from build123d import *

# Parameters (mm, degrees)
SKETCH1_R           = 1.5
SKETCH1_R_2         = 1
SKETCH1_R_3         = 0.5
BOSS_EXTRUDE1_DEPTH = 1.6
BOSS_EXTRUDE2_START = 1.6
SKETCH2_W           = 8
SKETCH2_H           = 8
BOSS_EXTRUDE2_DEPTH = 4.4
SKETCH3_W           = 10
SKETCH3_H           = 2.75
BOSS_EXTRUDE3_DEPTH = 3
SKETCH4_W           = 6.75
SKETCH4_H           = 6.75
SKETCH4_W_2         = 3
SKETCH4_H_2         = 3
SKETCH4_H_3         = 4
SKETCH4_W_3         = 1.5
BOSS_EXTRUDE4_DEPTH = 1.5


with BuildPart() as part:
    # Sketch1 → Boss-Extrude1 (new body)
    with BuildSketch(Plane(origin=(0, 0, 0), x_dir=(1, 0, 0), z_dir=(0, 1, 0))):
        with BuildLine():
            Line((-10, 28), (-10, 27))
            ThreePointArc((-10, 27), (-10.585786438, 25.585786438), (-12, 25))
            Line((-12, 25), (-15, 25))
            ThreePointArc((-15, 25), (-22.071067812, 22.071067812), (-25, 15))
            Line((-25, 15), (-25, -15))
            ThreePointArc((-25, -15), (-22.071067812, -22.071067812), (-15, -25))
            Line((-15, -25), (15, -25))
            ThreePointArc((15, -25), (22.071067812, -22.071067812), (25, -15))
            Line((25, -15), (25, 15))
            ThreePointArc((25, 15), (22.071067812, 22.071067812), (15, 25))
            Line((15, 25), (12, 25))
            ThreePointArc((12, 25), (10.585786438, 25.585786438), (10, 27))
            Line((10, 27), (10, 28))
            ThreePointArc((10, 28), (9.414213562, 29.414213562), (8, 30))
            Line((8, 30), (6, 30))
            Line((6, 30), (6, 27))
            ThreePointArc((6, 27), (4, 25), (2, 27))
            Line((2, 27), (2, 30))
            Line((2, 30), (-2, 30))
            Line((-2, 30), (-2, 27))
            ThreePointArc((-2, 27), (-4, 25), (-6, 27))
            Line((-6, 27), (-6, 30))
            Line((-6, 30), (-8, 30))
            ThreePointArc((-8, 30), (-9.414213562, 29.414213562), (-10, 28))
        make_face()
        with Locations((15.25, -15.25)):
            Circle(SKETCH1_R, mode=Mode.SUBTRACT)
        with Locations((-15.25, -15.25)):
            Circle(SKETCH1_R, mode=Mode.SUBTRACT)
        with Locations((-15.25, 15.25)):
            Circle(SKETCH1_R, mode=Mode.SUBTRACT)
        with Locations((15.25, 15.25)):
            Circle(SKETCH1_R, mode=Mode.SUBTRACT)
        with Locations((22, 12.5)):
            Circle(SKETCH1_R_2, mode=Mode.SUBTRACT)
        with Locations((22, -12.5)):
            Circle(SKETCH1_R_2, mode=Mode.SUBTRACT)
        with Locations((12.5, -22)):
            Circle(SKETCH1_R_2, mode=Mode.SUBTRACT)
        with Locations((-12.5, -22)):
            Circle(SKETCH1_R_2, mode=Mode.SUBTRACT)
        with Locations((-22, -12.5)):
            Circle(SKETCH1_R_2, mode=Mode.SUBTRACT)
        with Locations((-22, 12.5)):
            Circle(SKETCH1_R_2, mode=Mode.SUBTRACT)
        with Locations((-12.5, 22)):
            Circle(SKETCH1_R_2, mode=Mode.SUBTRACT)
        with Locations((12.5, 22)):
            Circle(SKETCH1_R_2, mode=Mode.SUBTRACT)
        with Locations((-1.25, -23.5)):
            Circle(SKETCH1_R_3, mode=Mode.SUBTRACT)
        with Locations((1.25, -23.5)):
            Circle(SKETCH1_R_3, mode=Mode.SUBTRACT)
        with Locations((-3.75, -23.5)):
            Circle(SKETCH1_R_3, mode=Mode.SUBTRACT)
        with Locations((-6.25, -23.5)):
            Circle(SKETCH1_R_3, mode=Mode.SUBTRACT)
        with Locations((-8.75, -23.5)):
            Circle(SKETCH1_R_3, mode=Mode.SUBTRACT)
        with Locations((3.75, -23.5)):
            Circle(SKETCH1_R_3, mode=Mode.SUBTRACT)
        with Locations((6.25, -23.5)):
            Circle(SKETCH1_R_3, mode=Mode.SUBTRACT)
        with Locations((8.75, -23.5)):
            Circle(SKETCH1_R_3, mode=Mode.SUBTRACT)
        with Locations((-8.75, -21)):
            Circle(SKETCH1_R_3, mode=Mode.SUBTRACT)
        with Locations((-6.25, -21)):
            Circle(SKETCH1_R_3, mode=Mode.SUBTRACT)
        with Locations((-3.75, -21)):
            Circle(SKETCH1_R_3, mode=Mode.SUBTRACT)
        with Locations((-1.25, -21)):
            Circle(SKETCH1_R_3, mode=Mode.SUBTRACT)
        with Locations((1.25, -21)):
            Circle(SKETCH1_R_3, mode=Mode.SUBTRACT)
        with Locations((3.75, -21)):
            Circle(SKETCH1_R_3, mode=Mode.SUBTRACT)
        with Locations((6.25, -21)):
            Circle(SKETCH1_R_3, mode=Mode.SUBTRACT)
        with Locations((8.75, -21)):
            Circle(SKETCH1_R_3, mode=Mode.SUBTRACT)
        with Locations((-21.01040764, -21.01040764)):
            Circle(SKETCH1_R_3, mode=Mode.SUBTRACT)
        with Locations((-19.001894566, -22.498989257)):
            Circle(SKETCH1_R_3, mode=Mode.SUBTRACT)
        with Locations((-22.498989257, -19.001894566)):
            Circle(SKETCH1_R_3, mode=Mode.SUBTRACT)
        with Locations((-19.001894566, 22.498989257)):
            Circle(SKETCH1_R_3, mode=Mode.SUBTRACT)
        with Locations((-21.01040764, 21.01040764)):
            Circle(SKETCH1_R_3, mode=Mode.SUBTRACT)
        with Locations((-22.498989257, 19.001894566)):
            Circle(SKETCH1_R_3, mode=Mode.SUBTRACT)
        with Locations((22.498989257, 19.001894566)):
            Circle(SKETCH1_R_3, mode=Mode.SUBTRACT)
        with Locations((21.01040764, 21.01040764)):
            Circle(SKETCH1_R_3, mode=Mode.SUBTRACT)
        with Locations((19.001894566, 22.498989257)):
            Circle(SKETCH1_R_3, mode=Mode.SUBTRACT)
        with Locations((19.001894566, -22.498989257)):
            Circle(SKETCH1_R_3, mode=Mode.SUBTRACT)
        with Locations((21.01040764, -21.01040764)):
            Circle(SKETCH1_R_3, mode=Mode.SUBTRACT)
        with Locations((22.498989257, -19.001894566)):
            Circle(SKETCH1_R_3, mode=Mode.SUBTRACT)
    extrude(amount=BOSS_EXTRUDE1_DEPTH)

    # Sketch2 → Boss-Extrude2 (add)
    with BuildSketch(Plane(origin=(0, 0, 0), x_dir=(1, 0, 0), z_dir=(0, 1, 0)).offset(BOSS_EXTRUDE2_START)):
        with Locations((-11.25, 8.5)):
            Rectangle(SKETCH2_W, SKETCH2_H)
        with Locations((11.25, -8.5)):
            Rectangle(SKETCH2_W, SKETCH2_H)
    extrude(amount=BOSS_EXTRUDE2_DEPTH)

    # Sketch3 → Boss-Extrude3 (add)
    with BuildSketch(Plane(origin=(0, 1.6, 0), x_dir=(1, 0, 0), z_dir=(0, 1, 0))):
        with Locations((0, -13.875)):
            Rectangle(SKETCH3_W, SKETCH3_H)
    extrude(amount=BOSS_EXTRUDE3_DEPTH)

    # Sketch4 → Boss-Extrude4 (add)
    with BuildSketch(Plane(origin=(0, 1.6, 0), x_dir=(1, 0, 0), z_dir=(0, 1, 0))):
        with Locations((-4.375, 18.625)):
            Rectangle(SKETCH4_W, SKETCH4_H)
        with Locations((4.375, 18.625)):
            Rectangle(SKETCH4_W, SKETCH4_H)
        with Locations((8.75, -2.5)):
            Rectangle(SKETCH4_W_2, SKETCH4_H_2)
        with Locations((9.25, 1.5)):
            Rectangle(SKETCH4_W_2, SKETCH4_H_3)
        with Locations((16.75, -4)):
            Rectangle(SKETCH4_W_3, SKETCH4_H_2)
        with Locations((-9.25, -1.5)):
            Rectangle(SKETCH4_W_2, SKETCH4_H_3)
        with Locations((16.75, 1)):
            Rectangle(SKETCH4_W_3, SKETCH4_H_2)
        with Locations((18.75, 1)):
            Rectangle(SKETCH4_W_3, SKETCH4_H_2)
        with Locations((18.75, -4)):
            Rectangle(SKETCH4_W_3, SKETCH4_H_2)
        with Locations((-8.75, 2.5)):
            Rectangle(SKETCH4_W_2, SKETCH4_H_2)
        with Locations((-16.75, -1)):
            Rectangle(SKETCH4_W_3, SKETCH4_H_2)
        with Locations((-18.75, -1)):
            Rectangle(SKETCH4_W_3, SKETCH4_H_2)
        with Locations((-16.75, 4)):
            Rectangle(SKETCH4_W_3, SKETCH4_H_2)
        with Locations((-18.75, 4)):
            Rectangle(SKETCH4_W_3, SKETCH4_H_2)
    extrude(amount=BOSS_EXTRUDE4_DEPTH)


solid = part.part
Read the model definition and answer for the solid it produces. Units are mm, in the model's axes. A direction names the side the tool comes from. Coordinates: 2 decimals unless noted, no trailing zeros. Loops run counter-clockwise (first coordinate to the right, second up) from the corner with the lowest first, then second, coordinate; pieces in that order, holes last.
Q1. The part is cut by section A-A on y = 5.2. Write down the section's boundary in (x, z).
Q2. Consider probe 1 along Z at (x, y) = (-12.5, 1.1); probe 2 along Z at (x, y) = (3.75, 1.25); probe 3 along Z at (x, y) = (2.5, 2.5). Determine where each line is inside the solid, lowest interval first.
Q3. Which of the six approach directions +Z, -Z, +X, -X, +Y, -Y give full straight-line access (tool end or side, diameter ignored) to faces 4 (the face through (7.25, 4, 9)), 5 (the face through (5, 3, 14)), 6 (the face through (-19.5, 2, -4)), 7 (the face through (-2, 1, -29))?
Q4. The part is cut by section B-B on y = 0.95. Give the number of separate pieces and of enclosed holes in the cut face, and give its area (3 significant figures).
Q5. Each of these flat-tipped pins is pushed along its axis until it touches: pin 1 Ø2.5 at (x, z) = (22, 12.5) entering from -Y; pin 2 Ø1.6 at (x, z) = (-22, 12.5) entering from -Y; pin 3 Ø2.5 at (x, z) = (9, -2) entering from +Y; pin 4 Ø0.5 at (y, z) = (1, -28) entering from -X. Where does it stop, or does it pass through?
Q6. The mould has two halves that part along X. Classify faces 1 (the face through (21.99, 0.79, 22.15)), 2 (the face through (-19, 2, -5.5)), 3 (the face through (16, 2, 4)): +X half, -X half, draft (parallel to the pull), parting line (faces both ways), or undercut.
Results below:
1. outline: (-15.25, -12.5) - (-7.25, -12.5) - (-7.25, -4.5) - (-15.25, -4.5) - close; (7.25, 4.5) - (15.25, 4.5) - (15.25, 12.5) - (7.25, 12.5) - close
2. probe 1: z = -25 to -23, -21 to 21, 23 to 25
2. probe 2: z = -25.02 to 20.5, 21.5 to 23, 24 to 25
2. probe 3: z = -22 to -15.25, 12.5 to 15.25
3. face 4: +Z, -X, +Y
3. face 5: +Z, +X, +Y
3. face 6: +Z, -Z, -X, +Y
3. face 7: -Z, +Y, -Y
4. separate pieces: 1
4. enclosed holes: 40
4. area: 2,400 mm2
5. pin 1: stops at y = 0
5. pin 2: passes through
5. pin 3: stops at y = 3.1
5. pin 4: stops at x = -10
6. face 1: +X half
6. face 2: draft
6. face 3: undercut
